from build123d import *

# Parameters (mm, degrees)
F0_W     = 75
F0_H     = 40
F0_W_2   = 69
F0_H_2   = 34
F1_DEPTH = 300
F2_W     = 40
F2_H     = 75
F2_W_2   = 34
F2_H_2   = 69
F3_DEPTH = 80
F4_R     = 5


with BuildPart() as f1:
    # F0 (on Top) → F1 (new body)
    with BuildSketch(Plane.XY):
        with Locations((-37.5, 20)):
            Rectangle(F0_W, F0_H)
        with Locations((-37.5, 20)):
            Rectangle(F0_W_2, F0_H_2, mode=Mode.SUBTRACT)
    extrude(amount=F1_DEPTH)

    # F2 (on face) → F3 (join)
    with BuildSketch(Plane(origin=(-75, 0, 0), x_dir=(0, -1, 0), z_dir=(-1, 0, 0))):
        with Locations((-20, 62.5)):
            Rectangle(F2_W, F2_H)
        with Locations((-20, 62.5)):
            Rectangle(F2_W_2, F2_H_2, mode=Mode.SUBTRACT)
    extrude(amount=F3_DEPTH)

    # F4
    f4_edges = [f1.edges().sort_by_distance(p)[0] for p in [
        (-75, 20, 100),
        (-75, 20, 25),
    ]]
    fillet(f4_edges, radius=F4_R)


solid = f1.part
Read the model definition and answer for the solid it produces. Units are mm, in the model's axes. A direction names the side the tool comes from. Give positions to 0.01 mm unless a question says otherwise; leave off trailing zeros. Write each loop counter-clockwise with the first axis right and the second up, starting at its lowest first coordinate (ties: lowest second). Pieces come first, ordered by that corner, then holes. Notation, with made-up numbers: M 89,80.5 L 128,80.5 A20 cw 128,89.5 Z; hole C 80,75 d7. An arc over 180 degrees is marked long. One line per item, written item: value. Start each with the question number.
(1) Find the intervals of material crossed by line 1 (X direction, y = 23.5, z = 172); line 2 (Y direction, x = -64.5, z = 259); line 3 (Z direction, x = -138, y = 15), in increasing order.
(2) Find section D-D (x = -116.5). Determine the outline of the cut face in (y, z).
(3) A tool of negligible diameter and unlimited length cuts with its end or side. For faces 5 (the flat face through (-114, 3, 62)), 6 (the flat face through (-75, 20, 10)), 7 (the flat face through (-72, 20, 148)), from which of +Z, -Z, +X, -X, +Y, -Y can it reach the whole face along a straight path? Write none if from no direction.
(4) Determine the mould class of faces 1 (the flat face through (-114, 20, 97)), 2 (the flat face through (0, 20, 148)), 3 (the flat face through (-44, 40, 115)), 4 (the flat face through (-3, 20, 148)) for opening direction Y: pulls with the +Y half, pulls with the -Y half, needs draft (parallel to the pull), parting line crosses it, or undercut.
(5) Find section C-C (y = 14.5). Determine the outline of the cut face in (x, z), plus the area to 3 significant figures.
(6) Find section A-A (x = -20). Determine the outline of the cut face in (y, z).
(7) Find section B-B (z = 148). Determine the outline of the cut face in (x, y), plus the area to 3 significant figures.
(8) Flat-ended cylindrical pins translate along their axes: pin 1 Ø12 at (y, z) = (29, 212) entering from -X; pin 2 Ø17 at (x, y) = (-131, 25) entering from -Z; pin 3 Ø10 at (x, y) = (-113, 16) entering from +Z. Find the tip coordinate at first contact, or state that the pin passes through.
Results below:
1. line 1: x = -75 to -72, -3 to 0
1. line 2: y = 0 to 3, 37 to 40
1. line 3: z = 25 to 28, 97 to 100
2. outline: M 0,25 L 40,25 L 40,100 L 0,100 Z; hole M 3,28 L 37,28 L 37,97 L 3,97 Z
3. face 5: -X
3. face 6: -Z, -X, +Y, -Y
3. face 7: +Z, -Z
4. face 1: undercut
4. face 2: needs draft
4. face 3: pulls with the +Y half
4. face 4: undercut
5. outline: M -155,25 L -80,25 A5 cw -75,20 L -75,0 L -72,0 L -72,300 L -75,300 L -75,105 A5 cw -80,100 L -155,100 L -155,97 L -75,97 L -75,28 L -155,28 Z; M -3,0 L 0,0 L 0,300 L -3,300 Z
5. area: 2,290 mm^2
6. outline: M 0,0 L 3,0 L 3,300 L 0,300 Z; M 37,0 L 40,0 L 40,300 L 37,300 Z
7. outline: M -75,0 L 0,0 L 0,40 L -75,40 Z; hole M -72,3 L -3,3 L -3,37 L -72,37 Z
7. area: 654 mm^2
8. pin 1: stops at x = -75
8. pin 2: stops at z = 25
8. pin 3: stops at z = 100
